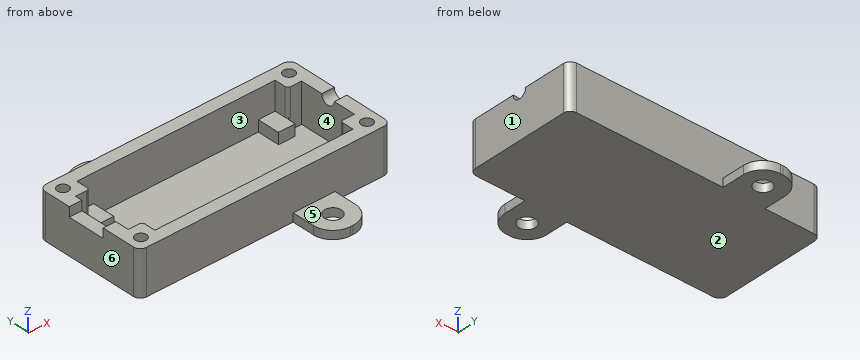
```python
from build123d import *

# Parameters (mm, degrees)
SKETCH_W        = 90
SKETCH_H        = 40
PAD_DEPTH       = 16
POCKET_DEPTH    = 14
POCKET001_DEPTH = 6
SKETCH003_W     = 13.5
SKETCH003_H     = 3.4
POCKET002_DEPTH = 6
SKETCH005_R     = 2
POCKET003_DEPTH = 10
SKETCH006_W     = 6
SKETCH006_H     = 8
PAD001_DEPTH    = 4
FILLET_R        = 2.5
FILLET001_R     = 1
SKETCH007_W     = 15
SKETCH007_H     = 3
PAD002_DEPTH    = 15
FILLET002_R     = 7
SKETCH008_R     = 3
HOLE_DEPTH      = 25
SKETCH009_W     = 15
SKETCH009_H     = 3
PAD003_DEPTH    = 15
FILLET003_R     = 7
SKETCH010_R     = 3
HOLE001_DEPTH   = 25


with BuildPart() as part:
    # Sketch → Pad (new body)
    with BuildSketch(Plane.XY):
        with Locations((45, 20)):
            Rectangle(SKETCH_W, SKETCH_H)
    extrude(amount=PAD_DEPTH)

    # Sketch001 (on Face6 of Pad) → Pocket (cut)
    with BuildSketch(Plane.XY.offset(16)):
        Polygon((4.5, 30.5), (4.5, 9.5), (9.5, 9.5), (9.5, 4.5), (80.5, 4.5), (80.5, 9.5), (85.5, 9.5), (85.5, 30.5), (80.5, 30.5), (80.5, 35.5), (9.5, 35.5), (9.5, 30.5), align=None)
    extrude(amount=-POCKET_DEPTH, mode=Mode.SUBTRACT)

    # Sketch002 (on Face6 of Pocket) → Pocket001 (cut)
    with BuildSketch(Plane.YZ.offset(90)):
        with BuildLine():
            ThreePointArc((17.5, 16), (20, 13.499987), (22.5, 16))
            Line((17.5, 16), (22.5, 16))
        make_face()
    extrude(amount=-POCKET001_DEPTH, mode=Mode.SUBTRACT)

    # Sketch003 (on Face1 of Pocket001) → Pocket002 (cut)
    with BuildSketch(Plane(origin=(0, 0, 0), x_dir=(0, -1, 0), z_dir=(-1, 0, 0))):
        with Locations((-21.25, 14.3)):
            Rectangle(SKETCH003_W, SKETCH003_H)
    extrude(amount=-POCKET002_DEPTH, mode=Mode.SUBTRACT)

    # Sketch005 (on Face8 of Pocket002) → Pocket003 (cut)
    with BuildSketch(Plane.XY.offset(16)):
        with Locations((4.5, 35.5)):
            Circle(SKETCH005_R)
        with Locations((4.5, 4.5)):
            Circle(SKETCH005_R)
        with Locations((85.5, 35.5)):
            Circle(SKETCH005_R)
        with Locations((85.5, 4.5)):
            Circle(SKETCH005_R)
    extrude(amount=-POCKET003_DEPTH, mode=Mode.SUBTRACT)

    # Sketch006 (on Face28 of Pocket003) → Pad001 (join)
    with BuildSketch(Plane.XY.offset(2)):
        with Locations((77.5, 31.5)):
            Rectangle(SKETCH006_W, SKETCH006_H)
        with Locations((12.5, 8.5)):
            Rectangle(SKETCH006_W, SKETCH006_H)
        with Locations((12.5, 31.5)):
            Rectangle(SKETCH006_W, SKETCH006_H)
        with Locations((77.5, 8.5)):
            Rectangle(SKETCH006_W, SKETCH006_H)
    extrude(amount=PAD001_DEPTH)

    # Fillet
    fillet_edges = [part.edges().sort_by_distance(p)[0] for p in [
        (0, 0, 8),
        (90, 0, 8),
        (90, 40, 8),
        (0, 40, 8),
    ]]
    fillet(fillet_edges, radius=FILLET_R)

    # Fillet001
    fillet001_edges = [part.edges().sort_by_distance(p)[0] for p in [
        (9.5, 30.5, 11),
        (80.5, 30.5, 11),
        (80.5, 9.5, 11),
        (9.5, 9.5, 11),
    ]]
    fillet(fillet001_edges, radius=FILLET001_R)

    # Sketch007 (on Face50 of Fillet001) → Pad002 (join)
    with BuildSketch(Plane.XZ):
        with Locations((62.5, 1.5)):
            Rectangle(SKETCH007_W, SKETCH007_H)
    extrude(amount=PAD002_DEPTH)

    # Fillet002
    fillet002_edges = [part.edges().sort_by_distance(p)[0] for p in [
        (55, -15, 1.5),
        (70, -15, 1.5),
    ]]
    fillet(fillet002_edges, radius=FILLET002_R)

    # Sketch008 (on Face8 of Fillet002) → Hole (cut)
    with BuildSketch(Plane.XY.offset(3)):
        with Locations((62.5, -7.5)):
            Circle(SKETCH008_R)
    extrude(amount=-HOLE_DEPTH, mode=Mode.SUBTRACT)

    # Sketch009 (on Face14 of Hole) → Pad003 (join)
    with BuildSketch(Plane(origin=(0, 40, 0), x_dir=(-1, 0, 0), z_dir=(0, 1, 0))):
        with Locations((-27.5, 1.5)):
            Rectangle(SKETCH009_W, SKETCH009_H)
    extrude(amount=PAD003_DEPTH)

    # Fillet003
    fillet003_edges = [part.edges().sort_by_distance(p)[0] for p in [
        (35, 55, 1.5),
        (20, 55, 1.5),
    ]]
    fillet(fillet003_edges, radius=FILLET003_R)

    # Sketch010 (on Face8 of Fillet003) → Hole001 (cut)
    with BuildSketch(Plane.XY.offset(3)):
        with Locations((27.5, 47.5)):
            Circle(SKETCH010_R)
    extrude(amount=-HOLE001_DEPTH, mode=Mode.SUBTRACT)


solid = part.part
```
Here's how the part is built. I have some questions about the finished solid (model axes, mm). Face numbers are marked on the shaded views. A direction names the side the tool comes from. Round coordinates to 2 decimals unless told otherwise and drop trailing zeros. Order: outer loops, then holes, each group sorted by start corner. A loop starts at its lowest first (then second) coordinate and runs counter-clockwise, first axis right, second up. Notation, with made-up numbers: M 61.25,-21.5 L 99.25,-21.5 A18 ccw 99.25,-12.5 Z; hole C 83.25,23.25 d11. An arc over 180 degrees is marked long. Answer in a Markdown table with one row per item.
Item 1: I'm going to push flat-ended pins straight in: pin 1 (6 mm diameter, centred on x = 16.5, y = 15.5, fed in from -Z); pin 2 (8 mm diameter, centred on x = 29, z = 11.5, fed in from -Y); pin 3 (1.5 mm diameter, centred on x = 76.5, z = 10, fed in from +Y); pin 4 (8 mm diameter, centred on x = 29.5, y = 26.5, fed in from +Z). Where does each tip first touch, or does it pass through?
A:
| item | result |
|---|---|
| pin 1 | stops at z = 0 |
| pin 2 | stops at y = 0 |
| pin 3 | stops at y = 40 |
| pin 4 | stops at z = 2 |
Item 2: For the marked faces 4, 5 and 6, which set-ups out of +Z, -Z, +X, -X, +Y, -Y let a thin tool reach every point of the face, with its end or its side?
A:
| item | result |
|---|---|
| face 4 | +Z |
| face 5 | +Z, +X, -X, -Y |
| face 6 | +Z, -Z, -X, +Y, -Y |
Item 3: Imagine slicing it at C-C, the plane z = 7.5. Write out the boundary of the cut face in (x, y), and give its area (3 significant figures).
A:
| item | result |
|---|---|
| outline | M 0,2.5 A2.5 ccw 2.5,0 L 87.5,0 A2.5 ccw 90,2.5 L 90,37.5 A2.5 ccw 87.5,40 L 2.5,40 A2.5 ccw 0,37.5 Z; hole C 4.5,4.5 d4; hole C 4.5,35.5 d4; hole M 4.5,9.5 L 8.5,9.5 A1 cw 9.5,8.5 L 9.5,4.5 L 80.5,4.5 L 80.5,8.5 A1 cw 81.5,9.5 L 85.5,9.5 L 85.5,30.5 L 81.5,30.5 A1 cw 80.5,31.5 L 80.5,35.5 L 9.5,35.5 L 9.5,31.5 A1 cw 8.5,30.5 L 4.5,30.5 Z; hole C 85.5,4.5 d4; hole C 85.5,35.5 d4 |
| area | 1,130 mm2 |
Item 4: Thinking about a two-plate mould opening in X: for the marked faces 1, 2 and 3, which applies, +X half, -X half, draft (parallel to the pull), parting line (faces both ways), or undercut?
A:
| item | result |
|---|---|
| face 1 | +X half |
| face 2 | draft |
| face 3 | undercut |
Item 5: Imagine slicing it at B-B, the plane y = 20. Write out the boundary of the cut face in (x, z), and give its area (3 significant figures).
A:
| item | result |
|---|---|
| outline | M 0,0 L 90,0 L 90,13.5 L 85.5,13.5 L 85.5,2 L 4.5,2 L 4.5,12.6 L 0,12.6 Z |
| area | 279 mm2 |
Item 6: Imagine slicing it at A-A, the plane x = 40.5. Write out the boundary of the cut face in (y, z), and give its area (3 significant figures).
A:
| item | result |
|---|---|
| outline | M 0,0 L 40,0 L 40,16 L 35.5,16 L 35.5,2 L 4.5,2 L 4.5,16 L 0,16 Z |
| area | 206 mm2 |
Item 7: Imagine slicing it at D-D, the plane x = 64. Write out the boundary of the cut face in (y, z).
A:
| item | result |
|---|---|
| outline | M -14.93,0 L -10.1,0 L -10.1,3 L -14.93,3 Z; M -4.9,0 L 40,0 L 40,16 L 35.5,16 L 35.5,2 L 4.5,2 L 4.5,16 L 0,16 L 0,3 L -4.9,3 Z |
Item 8: If I drill on L1, parallel to Y at x = 62.5, z = 2.35; L2, parallel to X at y = 20.5, z = 12; L3, parallel to Y at x = 18.5, z = 14.25, over which ranges is the centre line in solid material (lowest first)? Write a range as from..to.
A:
| item | result |
|---|---|
| L1 | y = -15..-10.5, -4.5..4.5, 35.5..40 |
| L2 | x = 0..4.5, 85.5..90 |
| L3 | y = 0..4.5, 35.5..40 |
